The model under review builds one solid part; all positions refer to its coordinate system, in mm. Face numbers are marked on the shaded views. Round coordinates to 2 decimals unless told otherwise and drop trailing zeros. Loops run counter-clockwise (first coordinate to the right, second up) from the corner with the lowest first, then second, coordinate; pieces in that order, holes last. Notation, with made-up numbers: M 20.25,11.25 L 34.25,11.25 A21 cw 34.25,46.25 Z; hole C -24.75,2.5 d3. An arc over 180 degrees is marked long. Answer as a JSON object with one key per item and string values. Group by question number.
Item 1: The part is to be moulded in two halves that separate along X. For the marked faces 1 and 2, say which applies: +X half, -X half, draft (parallel to the pull), parting line (faces both ways), or undercut.
Item 2: Consider section A-A (z = 10.5). Give the boundary of the cut face in (x, y).
Item 3: Consider section B-B (z = -62.5). Give the boundary of the cut face in (x, y), and give its area (3 significant figures).
Item 4: To check wall thickness, follow line 1 (Y direction, x = 18.2, z = -145.25); line 2 (X direction, y = -3.5, z = -33.5); line 3 (Y direction, x = 18, z = -100). State the ranges of each line that lie inside material, in increasing order.
Item 5: Consider section C-C (x = -2). Give the boundary of the cut face in (y, z).
Item 6: Insertion check: P1, Ø1.5, axis at x = -12, z = 81, coming from the +Y side; P2, Ø4.5, axis at y = 5.78, z = -145.25, coming from the -X side. Each pin has a flat end and moves straight along its axis. Give the tip position at first contact, or say it passes through.
```python
from build123d import *

# Parameters (mm, degrees)
BOSS_EXTRUDE1_DEPTH = 150
SKETCH2_R           = 1.75
SKETCH2_R_2         = 2.5
CUT_EXTRUDE1_DEPTH  = 156.283289507


with BuildPart() as part:
    # Sketch1 → Boss-Extrude1 (new, symmetric)
    with BuildSketch(Plane.XY):
        Polygon((-19.05, 12.7), (-17.4875, 12.7), (-17.4875, -11.1375), (17.4875, -11.1375), (17.4875, 12.7), (19.05, 12.7), (19.05, -12.7), (-19.05, -12.7), align=None)
    extrude(amount=BOSS_EXTRUDE1_DEPTH, both=True)

    # Sketch2 → Cut-Extrude1 (cut, through all)
    with BuildSketch(Plane(origin=(19.05, 0, 0), x_dir=(0, 0, -1), z_dir=(1, 0, 0))):
        with Locations(Location((145.25, 5.78125, 0), (0, 0, 90))):
            Circle(SKETCH2_R)
        with Locations(Location((145.25, -4.21875, 0), (0, 0, 90))):
            Circle(SKETCH2_R)
        with Locations(Location((-86, -0.1375, 0), (0, 0, 90))):
            Circle(SKETCH2_R_2)
        with Locations(Location((-126, 2.7, 0), (0, 0, 90))):
            Circle(SKETCH2_R_2)
        with Locations(Location((-60.5, 2.7, 0), (0, 0, 90))):
            Circle(SKETCH2_R_2)
        with Locations(Location((-71.25, 2.7, 0), (0, 0, 90))):
            Circle(SKETCH2_R)
        with Locations(Location((-49.75, 2.7, 0), (0, 0, 90))):
            Circle(SKETCH2_R)
        with Locations(Location((-21.25, 2.7, 0), (0, 0, 90))):
            Circle(SKETCH2_R)
        with Locations(Location((-10.5, 2.7, 0), (0, 0, 90))):
            Circle(SKETCH2_R_2)
        with Locations(Location((0.25, 2.7, 0), (0, 0, 90))):
            Circle(SKETCH2_R)
        with Locations(Location((28.75, 2.7, 0), (0, 0, 90))):
            Circle(SKETCH2_R)
        with Locations(Location((39.5, 2.7, 0), (0, 0, 90))):
            Circle(SKETCH2_R_2)
        with Locations(Location((50.25, 2.7, 0), (0, 0, 90))):
            Circle(SKETCH2_R)
        with Locations(Location((78.75, 2.7, 0), (0, 0, 90))):
            Circle(SKETCH2_R)
        with Locations(Location((89.5, 2.7, 0), (0, 0, 90))):
            Circle(SKETCH2_R_2)
        with Locations(Location((100.25, 2.7, 0), (0, 0, 90))):
            Circle(SKETCH2_R)
    extrude(amount=-CUT_EXTRUDE1_DEPTH, mode=Mode.SUBTRACT)


solid = part.part
```
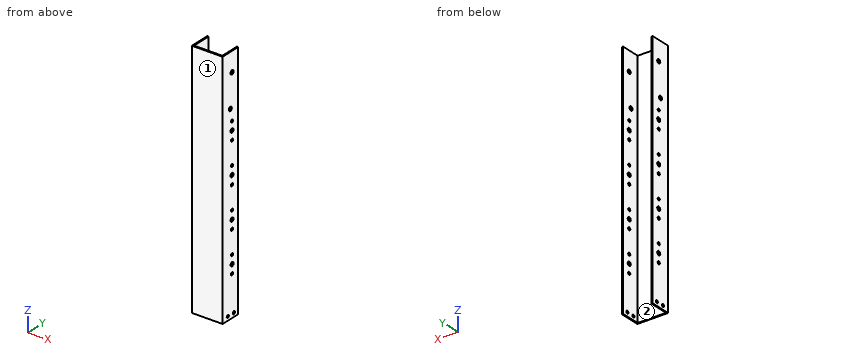
Geometry results:
{
 "1": {"face 1": "draft", "face 2": "undercut"},
 "2": {"outline": "M -19.05,-12.7 L 19.05,-12.7 L 19.05,0.2 L 17.49,0.2 L 17.49,-11.14 L -17.49,-11.14 L -17.49,0.2 L -19.05,0.2 Z; M -19.05,5.2 L -17.49,5.2 L -17.49,12.7 L -19.05,12.7 Z; M 17.49,5.2 L 19.05,5.2 L 19.05,12.7 L 17.49,12.7 Z"},
 "3": {"outline": "M -19.05,-12.7 L 19.05,-12.7 L 19.05,12.7 L 17.49,12.7 L 17.49,-11.14 L -17.49,-11.14 L -17.49,12.7 L -19.05,12.7 Z", "area": "134 mm^2"},
 "4": {"line 1": "y = -12.7 to -5.97, -2.47 to 4.03, 7.53 to 12.7", "line 2": "x = -19.05 to -17.49, 17.49 to 19.05", "line 3": "y = -12.7 to 0.97, 4.43 to 12.7"},
 "5": {"outline": "M -12.7,-150 L -11.14,-150 L -11.14,150 L -12.7,150 Z"},
 "6": {"P1": "stops at y = -11.14", "P2": "stops at x = -19.05"}
}
